from build123d import *

# Parameters (mm, degrees)
SKETCH1_W             = 8
SKETCH1_H             = 12
SKETCH1_R             = 2
BOSS_EXTRUDE1_DEPTH   = 2.5
BOSS_EXTRUDE1_2_DEPTH = 2.5
BOSS_EXTRUDE1_3_DEPTH = 2.5
SKETCH2_W             = 8
SKETCH2_H             = 3
BOSS_EXTRUDE2_DEPTH   = 30
SKETCH3_R             = 1.75
SKETCH3_W             = 12.333333333
SKETCH3_H             = 21
SKETCH3_W_2           = 12.333333334
BOSS_EXTRUDE3_DEPTH   = 2.5
FILLET1_R             = 3
FILLET2_R             = 4
FILLET3_R             = 2
FILLET4_R             = 2


with BuildPart() as part:
    # Sketch1 → Boss-Extrude1 (new body)
    with BuildSketch(Plane(origin=(0, 0, 0), x_dir=(1, 0, 0), z_dir=(0, 1, 0))):
        with Locations((-41, 78)):
            Rectangle(SKETCH1_W, SKETCH1_H)
        with Locations(Location((-41, 80, 0), (0, 0, 270))):
            Circle(SKETCH1_R, mode=Mode.SUBTRACT)
    extrude(amount=BOSS_EXTRUDE1_DEPTH)



with BuildPart() as body_2:
    # Sketch1 → Boss-Extrude1 2 (new body)
    with BuildSketch(Plane(origin=(0, 0, 0), x_dir=(1, 0, 0), z_dir=(0, 1, 0))):
        with Locations((4, -6)):
            Rectangle(SKETCH1_W, SKETCH1_H)
        with Locations(Location((4, -8, 0), (0, 0, 270))):
            Circle(SKETCH1_R, mode=Mode.SUBTRACT)
    extrude(amount=BOSS_EXTRUDE1_2_DEPTH)


with BuildPart() as body_3:
    # Sketch1 → Boss-Extrude1 3 (new body)
    with BuildSketch(Plane(origin=(0, 0, 0), x_dir=(1, 0, 0), z_dir=(0, 1, 0))):
        with Locations((4, 78)):
            Rectangle(SKETCH1_W, SKETCH1_H)
        with Locations(Location((4, 80, 0), (0, 0, 270))):
            Circle(SKETCH1_R, mode=Mode.SUBTRACT)
    extrude(amount=BOSS_EXTRUDE1_3_DEPTH)


with BuildPart() as part_1:
    add(part.part)

    add(body_2.part)  # Boss-Extrude2 merges body 2

    add(body_3.part)  # Boss-Extrude2 merges body 3
    # Sketch2 → Boss-Extrude2 (add)
    with BuildSketch(Plane(origin=(0, 2.5, 0), x_dir=(1, 0, 0), z_dir=(0, 1, 0))):
        with Locations((-41, 73.5)):
            Rectangle(SKETCH2_W, SKETCH2_H)
        with Locations((4, 73.5)):
            Rectangle(SKETCH2_W, SKETCH2_H)
        with Locations((4, -1.5)):
            Rectangle(SKETCH2_W, SKETCH2_H)
    extrude(amount=BOSS_EXTRUDE2_DEPTH)

    # Sketch3 → Boss-Extrude3 (add)
    with BuildSketch(Plane(origin=(0, 32.5, 0), x_dir=(1, 0, 0), z_dir=(0, 1, 0))):
        Polygon((-45, 75), (8, 75), (8, -3), (-7, -3), (-7, 15), (-45, 15), align=None)
        with Locations(Location((4, 5, 0), (0, 0, 270))):
            Circle(SKETCH3_R, mode=Mode.SUBTRACT)
        with Locations(Location((4, 17, 0), (0, 0, 270))):
            Circle(SKETCH3_R, mode=Mode.SUBTRACT)
        with Locations((-34.833333334, 58.5)):
            Rectangle(SKETCH3_W, SKETCH3_H, mode=Mode.SUBTRACT)
        with Locations((-18.5, 58.5)):
            Rectangle(SKETCH3_W_2, SKETCH3_H, mode=Mode.SUBTRACT)
        with Locations((-2.166666667, 58.5)):
            Rectangle(SKETCH3_W, SKETCH3_H, mode=Mode.SUBTRACT)
        with Locations((-34.833333334, 31.5)):
            Rectangle(SKETCH3_W, SKETCH3_H, mode=Mode.SUBTRACT)
        with Locations((-18.5, 31.5)):
            Rectangle(SKETCH3_W_2, SKETCH3_H, mode=Mode.SUBTRACT)
        with Locations((-2.166666667, 31.5)):
            Rectangle(SKETCH3_W, SKETCH3_H, mode=Mode.SUBTRACT)
    extrude(amount=BOSS_EXTRUDE3_DEPTH)

    # Fillet1
    fillet1_edges = [part_1.edges().sort_by_distance(p)[0] for p in [
        (-24.666666667, 33.75, -48),
        (-12.333333333, 33.75, -48),
        (-12.333333333, 33.75, -69),
        (-24.666666667, 33.75, -69),
        (-41, 33.75, -48),
        (-28.666666667, 33.75, -48),
        (-28.666666667, 33.75, -69),
        (-41, 33.75, -69),
        (-8.333333333, 33.75, -48),
        (4, 33.75, -48),
        (4, 33.75, -69),
        (-8.333333333, 33.75, -69),
        (-41, 33.75, -21),
        (-28.666666667, 33.75, -21),
        (-28.666666667, 33.75, -42),
        (-41, 33.75, -42),
        (-24.666666667, 33.75, -21),
        (-12.333333333, 33.75, -21),
        (-12.333333333, 33.75, -42),
        (-24.666666667, 33.75, -42),
        (-8.333333333, 33.75, -21),
        (4, 33.75, -21),
        (4, 33.75, -42),
        (-8.333333333, 33.75, -42),
    ]]
    fillet(fillet1_edges, radius=FILLET1_R)

    # Fillet2
    fillet2_edges = [part_1.edges().sort_by_distance(p)[0] for p in [
        (-45, 33.75, -15),
        (-7, 33.75, -15),
        (-7, 33.75, 3),
    ]]
    fillet(fillet2_edges, radius=FILLET2_R)

    # Fillet3
    fillet3_edges = [part_1.edges().sort_by_distance(p)[0] for p in [
        (4, 2.5, 3),
        (4, 2.5, -75),
        (-41, 2.5, -75),
    ]]
    fillet(fillet3_edges, radius=FILLET3_R)

    # Fillet4
    fillet4_edges = [part_1.edges().sort_by_distance(p)[0] for p in [
        (4, 32.5, 0),
        (4, 32.5, -72),
        (-41, 32.5, -72),
    ]]
    fillet(fillet4_edges, radius=FILLET4_R)


solid = part_1.part
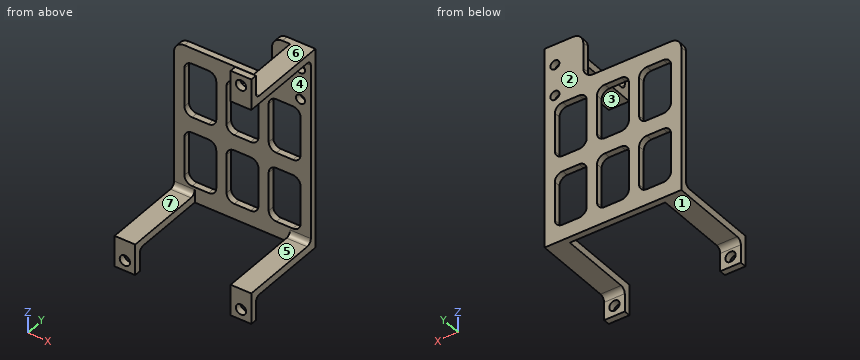
Can you work these out from the model? Positions are in its coordinate system, mm. Face numbers are marked on the shaded views. A direction names the side the tool comes from. Round coordinates to 2 decimals unless told otherwise and drop trailing zeros. Write each loop counter-clockwise with the first axis right and the second up, starting at its lowest first coordinate (ties: lowest second). Pieces come first, ordered by that corner, then holes. Notation, with made-up numbers: (88, -19) -> (145, -19) arc R11 cw to (145, -10) -> close; hole circle Ø7 at (42.5, 14). An arc over 180 degrees is marked (long way). Use one line per item in the form item = value. Start each with the question number.
Q1. Imagine slicing it at C-C (z = -5). Please give me the cut outline in (x, y).
Q2. Which directions (+Z, -Z, +X, -X, +Y, -Y) give clear straight access to the entire face, cutting with the end or side of a thin tool? Please do the marked faces 4, 5, 6 and 7.
Q3. We'd pull the mould along Z, two halves only. Please class the marked faces 1, 2 and 3: +Z half, -Z half, draft (parallel to the pull), parting line (faces both ways), or undercut.
Q4. Imagine slicing it at A-A (y = 13). Please give me the cut outline in (x, z).
Q5. Imagine slicing it at B-B (z = -80). Please give me the cut outline in (x, y), then the cut area to 3 significant figures.
Q6. I'm going to push flat-ended pins straight in: P1, Ø0.8, axis at y = 34.5, z = -8, coming from the -X side; P2, Ø0.8, axis at x = -17.5, y = 34, coming from the +Z side; P3, Ø7.5, axis at x = 4.5, z = -79, coming from the +Y side. Where does each tip first touch, or does it pass through?
Q7. If I drill on probe 1 along X at (y, z) = (0.65, -80); probe 2 along Z at (x, y) = (-15, 33); probe 3 along Z at (x, y) = (5.5, 26), over which ranges is the centre line in solid material (lowest first)? Write a range as [from, to].
Q8. Imagine slicing it at D-D (x = -16.5). Please give me the cut outline in (y, z), then the cut area to 3 significant figures.
Worked out:
q1.outline = (-7, 32.5) -> (2.25, 32.5) -> (2.25, 35) -> (-7, 35) -> close; (5.75, 32.5) -> (8, 32.5) -> (8, 35) -> (5.75, 35) -> close
q2.face_4 = -Y
q2.face_5 = +X, -X, -Y
q2.face_6 = +Z, +X, -X, +Y
q2.face_7 = +Z, +X, -X, -Y
q3.face_1 = -Z half
q3.face_2 = draft
q3.face_3 = undercut
q4.outline = (-45, -75) -> (-37, -75) -> (-37, -72) -> (-45, -72) -> close; (0, -75) -> (8, -75) -> (8, -72) -> (0, -72) -> close; (0, 0) -> (8, 0) -> (8, 3) -> (0, 3) -> close
q5.outline = (-45, 0) -> (-43, 0) -> (-43, 2.5) -> (-45, 2.5) -> close; (-39, 0) -> (-37, 0) -> (-37, 2.5) -> (-39, 2.5) -> close; (0, 0) -> (2, 0) -> (2, 2.5) -> (0, 2.5) -> close; (6, 0) -> (8, 0) -> (8, 2.5) -> (6, 2.5) -> close
q5.area = 20.0 mm^2
q6.P1 = -7
q6.P2 = -15
q6.P3 = 3.53
q7.probe_1 = [-45, -43], [-39, -37], [0, 2], [6, 8]
q7.probe_2 = [-75, -68.98], [-48.02, -41.98], [-21.02, -15]
q7.probe_3 = [-75, -72], [0, 3]
q8.outline = (32.5, -75) -> (35, -75) -> (35, -69) -> (32.5, -69) -> close; (32.5, -48) -> (35, -48) -> (35, -42) -> (32.5, -42) -> close; (32.5, -21) -> (35, -21) -> (35, -15) -> (32.5, -15) -> close
q8.area = 45.0 mm^2
